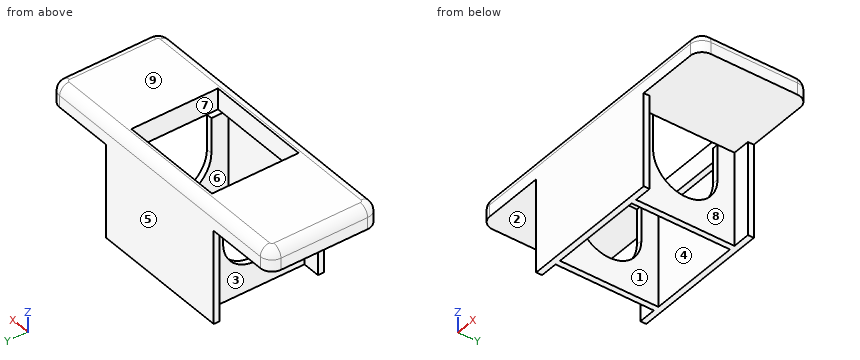
```python
from build123d import *

# Parameters (mm, degrees)
SKETCH001_W     = 24.4
SKETCH001_H     = 9.4
PAD_DEPTH       = 1.8
SKETCH_W        = 8
SKETCH_H        = 8.4
PAD001_DEPTH    = 8
SKETCH002_W     = 9
SKETCH002_H     = 7.4
POCKET_DEPTH    = 1.8
POCKET002_DEPTH = 16.701
FILLET_R        = 1
FILLET001_R     = 0.8


with BuildPart() as part:
    # Sketch001 → Pad (new body)
    with BuildSketch(Plane.XY):
        with Locations((12.2, 4.7)):
            Rectangle(SKETCH001_W, SKETCH001_H)
    extrude(amount=PAD_DEPTH)

    # Sketch (on Face5 of Pad) → Pad001 (join)
    with BuildSketch(Plane(origin=(0, 0, 0), x_dir=(1, 0, 0), z_dir=(0, 0, -1))):
        Polygon((6.2, 0), (6.2, -0.5), (7.7, -0.5), (7.7, -8.9), (6.2, -8.9), (6.2, -9.4), (18.2, -9.4), (18.2, -8.9), (16.7, -8.9), (16.7, -0.5), (18.2, -0.5), (18.2, 0), align=None)
        with Locations((12.2, -4.7)):
            Rectangle(SKETCH_W, SKETCH_H, mode=Mode.SUBTRACT)
    extrude(amount=PAD001_DEPTH)

    # Sketch002 (on Face25 of Pad001) → Pocket (cut)
    with BuildSketch(Plane(origin=(0, 0, 0), x_dir=(1, 0, 0), z_dir=(0, 0, -1))):
        with Locations((12.2, -4.7)):
            Rectangle(SKETCH002_W, SKETCH002_H)
    extrude(amount=-POCKET_DEPTH, mode=Mode.SUBTRACT)

    # Sketch004 → Pocket002 (cut, through all)
    with BuildSketch(Plane(origin=(7.7, 0, 0), x_dir=(0, -1, 0), z_dir=(-1, 0, 0))):
        with BuildLine():
            Line((-7.45, -3), (-7.45, 0))
            Line((-7.45, 0), (-1.95, 0))
            Line((-1.95, 0), (-1.95, -3))
            ThreePointArc((-7.45, -3), (-4.7, -5.75), (-1.95, -3))
        make_face()
    extrude(amount=-POCKET002_DEPTH, mode=Mode.SUBTRACT)

    # Fillet
    fillet_edges = [part.edges().sort_by_distance(p)[0] for p in [
        (0, 0, 0.9),
        (0, 9.4, 0.9),
        (24.4, 0, 0.9),
        (24.4, 9.4, 0.9),
    ]]
    fillet(fillet_edges, radius=FILLET_R)

    # Fillet001
    fillet001_edges = [part.edges().sort_by_distance(p)[0] for p in [
        (0.292893, 0.292893, 1.8),
        (0, 4.7, 1.8),
        (0.292893, 9.107107, 1.8),
        (12.2, 9.4, 1.8),
        (24.107107, 9.107107, 1.8),
        (24.4, 4.7, 1.8),
        (24.107107, 0.292893, 1.8),
        (12.2, 0, 1.8),
    ]]
    fillet(fillet001_edges, radius=FILLET001_R)


solid = part.part
```
Check sheet for the modelled part. Datum: model origin and axes. Units: mm. Face numbers are marked on the shaded views. A direction names the side the tool comes from. Round coordinates to 2 decimals unless told otherwise and drop trailing zeros. Write each loop counter-clockwise with the first axis right and the second up, starting at its lowest first coordinate (ties: lowest second). Pieces come first, ordered by that corner, then holes. Notation, with made-up numbers: (-26.75, 10) -> (-16.75, 10) arc R27 ccw to (-16.75, 34) -> close; hole circle Ø8 at (27.5, 22). An arc over 180 degrees is marked (long way). One line per question, with ' | ' between items. Start each with the question number.
1. Depth check by flat-ended pin: pin 1 (2.5 mm diameter, centred on y = 4, z = -4, fed in from +X); pin 2 (2.5 mm diameter, centred on x = 4.5, y = 7, fed in from -Z). Enter the tip coordinate at first touch or a pass-through.
2. Release check for a two-part mould opening along X. For the marked faces 1, 2, 3 and 4 record: +X half, -X half, draft (parallel to the pull), parting line (faces both ways), or undercut.
3. Sectioned sample at C-C, the plane z = 0.25. Record the cut outline in (x, y).
4. Sectioned sample at D-D, the plane x = 4.75. Record the cut outline in (y, z), then the cut area to 3 significant figures.
5. Set-up check for the marked faces 5, 6, 7, 8 and 9: record each of +Z, -Z, +X, -X, +Y, -Y from which the full face is reachable in a straight line by a thin tool's end or side.
6. Scan lines: line 1 along X through (y, z) = (2.25, -5); line 2 along Y through (x, z) = (12.5, -1); line 3 along Y through (x, z) = (16.5, -1.25). Record each from-to range of solid material in increasing order. Write a range as from..to.
7. Sectioned sample at A-A, the plane z = -2.5. Record the cut outline in (x, y).
Taken from the geometry:
1) pin 1: passes through | pin 2: stops at z = 0
2) face 1: undercut | face 2: draft | face 3: -X half | face 4: undercut
3) outline: (0, 1) arc R1 ccw to (1, 0) -> (23.4, 0) arc R1 ccw to (24.4, 1) -> (24.4, 8.4) arc R1 ccw to (23.4, 9.4) -> (1, 9.4) arc R1 ccw to (0, 8.4) -> close; hole (7.7, 1) -> (16.7, 1) -> (16.7, 8.4) -> (7.7, 8.4) -> close
4) outline: (0, 0) -> (9.4, 0) -> (9.4, 1) arc R0.8 ccw to (8.6, 1.8) -> (0.8, 1.8) arc R0.8 ccw to (0, 1) -> close | area: 16.6 mm^2
5) face 5: +Z, -Z, +X, -X, +Y | face 6: -Z | face 7: +Z | face 8: -Z, +X | face 9: +Z, +X, -X, +Y, -Y
6) line 1: x = 7.7..8.2, 16.2..16.7 | line 2: y = 0..0.5, 8.9..9.4 | line 3: y = 0..1.95, 7.45..9.4
7) outline: (6.2, 0) -> (18.2, 0) -> (18.2, 0.5) -> (16.7, 0.5) -> (16.7, 1.95) -> (16.2, 1.95) -> (16.2, 0.5) -> (8.2, 0.5) -> (8.2, 1.95) -> (7.7, 1.95) -> (7.7, 0.5) -> (6.2, 0.5) -> close; (6.2, 8.9) -> (7.7, 8.9) -> (7.7, 7.45) -> (8.2, 7.45) -> (8.2, 8.9) -> (16.2, 8.9) -> (16.2, 7.45) -> (16.7, 7.45) -> (16.7, 8.9) -> (18.2, 8.9) -> (18.2, 9.4) -> (6.2, 9.4) -> close
